Check sheet for the drawn part. Datum: minimum x, y, z corner. Units: mm. Round coordinates to 2 decimals unless told otherwise and drop trailing zeros. One line per item, written item: value. Start each with the question number.
Item 1: Thickness scan on probe 1 along X at (y, z) = (0.7, 10.5) (1 decimal); probe 2 along X at (y, z) = (1.15, 9) (1 decimal); probe 3 along Z at (x, y) = (6.75, 2). Record the ranges inside material, lowest first. Write a range as from..to.
Item 2: Draft check along Z on the marked faces 1, 2, 3 and 4. Enter one of: +Z half, -Z half, draft (parallel to the pull), parting line (faces both ways), or undercut.
Item 3: Gauge pin test, flat ends, axial feed: pin 1 (1.5 mm diameter, centred on x = 2, y = 0.5, fed in from +Z) (1 decimal); pin 2 (1.5 mm diameter, centred on x = 8.5, z = 12, fed in from -Y); pin 3 (1 mm diameter, centred on y = 0.5, z = 8, fed in from +X). Record the tip position at first contact, or that the pin passes through.
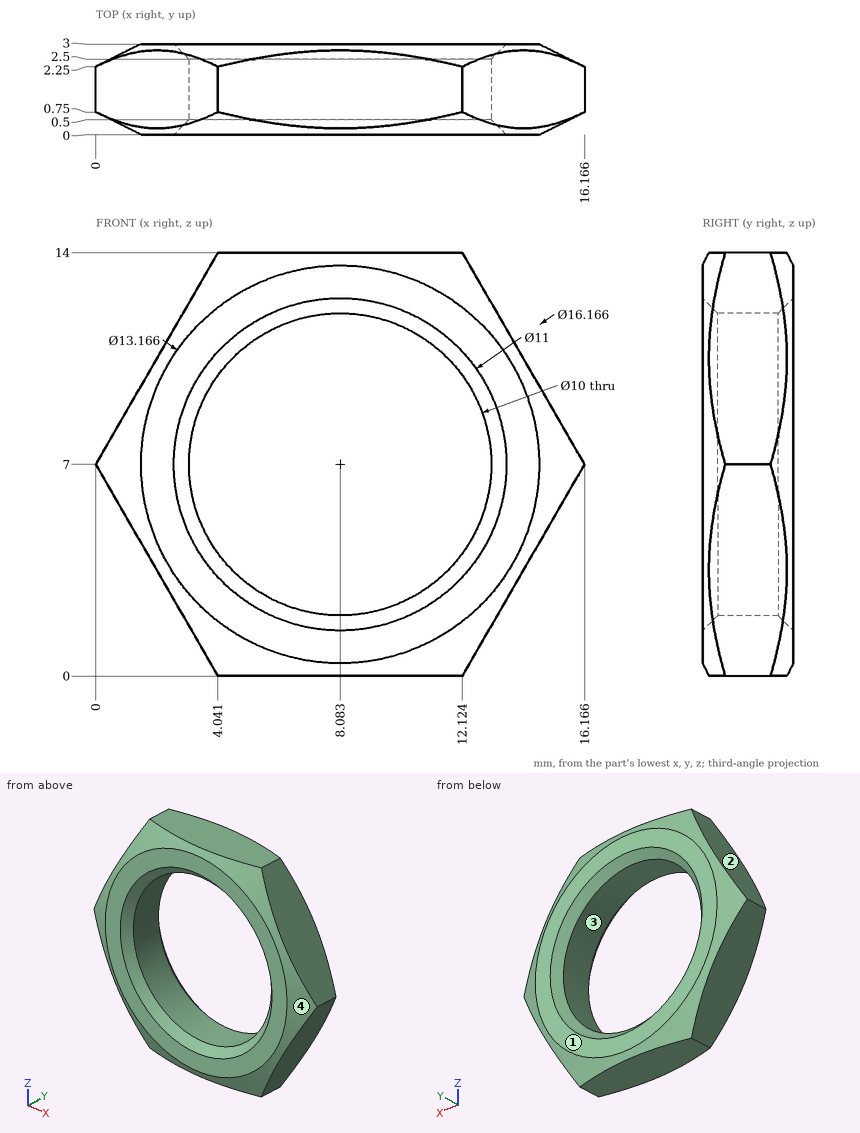
Response values:
1. probe 1: x = 2..4.5, 11.7..14.1
1. probe 2: x = 1.2..3.5, 12.7..15
1. probe 3: z = 0..2.18, 11.82..14
2. face 1: draft
2. face 2: +Z half
2. face 3: undercut
2. face 4: parting line
3. pin 1: stops at z = 11.8
3. pin 2: stops at y = 0
3. pin 3: stops at x = 15.87
